Here's how the part is built. I have some questions about the finished solid (model axes, mm). A direction names the side the tool comes from. Coordinates: 2 decimals unless noted, no trailing zeros. Write each loop counter-clockwise with the first axis right and the second up, starting at its lowest first coordinate (ties: lowest second). Pieces come first, ordered by that corner, then holes. Notation, with made-up numbers: (52, 38) -> (102, 38) arc R24 cw to (102, 61) -> close; hole circle Ø6 at (43.5, 42.5). An arc over 180 degrees is marked (long way). Put each result on its own line as item: value. Start each with the question number.
Item 1: I need wall thicknesses on line 1 (Y direction, x = 0, z = 1.9); line 2 (Y direction, x = 15.5, z = 1.2); line 3 (Y direction, x = 22.5, z = 2.05). Which ranges of each line are inside material? Lowest first, please. Write a range as [from, to].
Item 2: On a 3-axis mill with a long thin cutter (end or side, diameter ignored), from which of +Z, -Z, +X, -X, +Y, -Y can I reach the whole of each face in a straight line? I mean faces 5 (the face through (25, 3, 3)), 6 (the face through (52.312, 6.722, 1.479)). Say none if no direction works.
Item 3: I want a section at B-B, the plane x = 5.5. List the corners of the cut face in (y, z) for me.
Item 4: I want a section at A-A, the plane z = 2.5. State how many separate pieces and enclosed holes the cut face has, then the cut area to 3 significant figures.
Item 5: I want a section at C-C, the plane y = 11. List the corners of the cut face in (x, z) for me, then the cut area to 3 significant figures.
Item 6: If we mould it in two halves opening along X, with no side actions, what happens to faces 1 (the face through (25, 3, 0)), 2 (the face through (33.17, 4.27, 1.48)), 3 (the face through (33.301, 10.448, 1.479)), 4 (the face through (54.561, 10.473, 1.479))? For each: released by +X, released by -X, zero draft, split by the parting line, or undercut.
Item 7: For pin 1 (5 mm diameter, centred on x = 46.5, y = 8, fed in from -Z); pin 2 (1.5 mm diameter, centred on y = 6, z = 1.5, fed in from -X); pin 3 (2.5 mm diameter, centred on x = 22.02, y = 0.21, fed in from -Z); pin 4 (1.5 mm diameter, centred on y = 11.5, z = 0.5, fed in from -X), each with a flat end and sliding along its axis, tell me the tip position at first contact or that it passes through.
from build123d import *

# Parameters (mm, degrees)
SKETCH1_R           = 1.5
BOSS_EXTRUDE3_DEPTH = 3
FILLET1_R           = 1


with BuildPart() as part:
    # Sketch1 → Boss-Extrude3 (new body)
    with BuildSketch(Plane.XY):
        with BuildLine():
            Line((20.05, 5), (0, 5))
            ThreePointArc((0, 5), (-5, 0), (0, -5))
            Line((0, -5), (22, -5))
            Line((22, -5), (26.72989842, 1.621129525))
            Line((26.72989842, 1.621129525), (39.900164389, 7.036080522))
            Line((39.900164389, 7.036080522), (46.188488025, 4.540007042))
            Line((46.188488025, 4.540007042), (47.352932204, 4.337597171))
            Line((47.352932204, 4.337597171), (48.038244482, 5.300533868))
            Line((48.038244482, 5.300533868), (49.20268866, 5.098123997))
            Line((49.20268866, 5.098123997), (49.888000938, 6.061060693))
            Line((49.888000938, 6.061060693), (51.052445116, 5.858650822))
            Line((51.052445116, 5.858650822), (51.737757394, 6.821587519))
            Line((51.737757394, 6.821587519), (52.902201573, 6.619177648))
            Line((52.902201573, 6.619177648), (53.587513851, 7.582114344))
            Line((53.587513851, 7.582114344), (54.751958029, 7.379704473))
            Line((54.751958029, 7.379704473), (55.437270307, 8.34264117))
            Line((55.437270307, 8.34264117), (53.72608495, 12.504593197))
            Line((53.72608495, 12.504593197), (46.409029503, 15.837507263))
            Line((46.409029503, 15.837507263), (20.05, 5))
        make_face()
        Circle(SKETCH1_R, mode=Mode.SUBTRACT)
        with Locations((22.020705275, 0.206842568)):
            Circle(SKETCH1_R, mode=Mode.SUBTRACT)
    extrude(amount=BOSS_EXTRUDE3_DEPTH)

    # Fillet1
    fillet1_edges = [part.edges().sort_by_distance(p)[0] for p in [
        (22, -5, 1.5),
        (20.05, 5, 1.5),
        (46.409029503, 15.837507263, 1.5),
        (53.72608495, 12.504593197, 1.5),
        (55.437270307, 8.34264117, 1.5),
        (46.188488025, 4.540007042, 1.5),
        (39.900164389, 7.036080522, 1.5),
        (26.72989842, 1.621129525, 1.5),
    ]]
    fillet(fillet1_edges, radius=FILLET1_R)


solid = part.part
Calculated:
1. line 1: y = [-5, -1.5], [1.5, 5]
1. line 2: y = [-5, 5]
1. line 3: y = [-4.3, -1.21], [1.63, 6.01]
2. face 5: +Z, +X, -X, +Y, -Y
2. face 6: +Z, -Z, -Y
3. outline: (-5, 0) -> (5, 0) -> (5, 3) -> (-5, 3) -> close
4. separate pieces: 1
4. enclosed holes: 2
4. area: 490 mm2
5. outline: (34.64, 0) -> (54.34, 0) -> (54.34, 3) -> (34.64, 3) -> close
5. area: 59.1 mm2
6. face 1: zero draft
6. face 2: undercut
6. face 3: released by -X
6. face 4: released by +X
7. pin 1: stops at z = 0
7. pin 2: stops at x = 20.66
7. pin 3: passes through
7. pin 4: stops at x = 34.04
